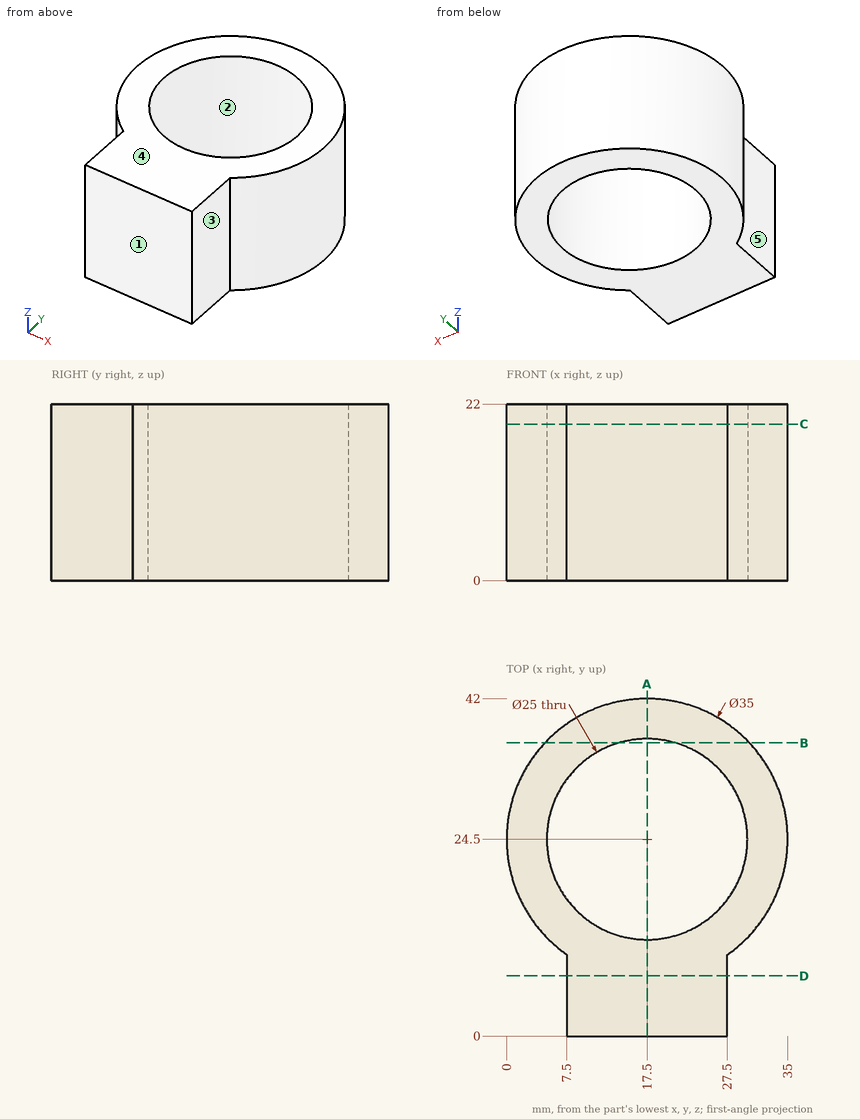
Verification items for this drawing (mm, ordinates from the low corner). A direction names the side the tool comes from. Coordinates: 2 decimals unless noted, no trailing zeros. Write each loop counter-clockwise with the first axis right and the second up, starting at its lowest first coordinate (ties: lowest second). Pieces come first, ordered by that corner, then holes. Notation, with made-up numbers: M 40.25,9 L 76.25,9 A14 ccw 76.25,17 Z; hole C 76,31 d10. An arc over 180 degrees is marked long. One line per item, written item: value. Start each with the question number.
(1) Sectioned sample at D-D, the plane y = 7.5. Enter the section's corners in (x, z).
(2) Sectioned sample at C-C, the plane z = 19.5. Enter the section's corners in (x, y).
(3) Tool access check on the marked faces 4 and 5. Record the directions out of +Z, -Z, +X, -X, +Y, -Y that give a thin tool (end or side, any length) a straight path to the whole face; none if there is none.
(4) Scan lines: line 1 along Y through (x, z) = (17.5, 17.5); line 2 along X through (y, z) = (2, 1.5); line 3 along Y through (x, z) = (21, 4.25). Record each from-to range of solid material in increasing order. Write a range as [from, to].
(5) Sectioned sample at A-A, the plane x = 17.5. Enter the section's corners in (y, z), and give its area (3 significant figures).
(6) Sectioned sample at B-B, the plane y = 36.5. Enter the section's corners in (x, z), and give its area (3 significant figures).
(7) Release check for a two-part mould opening along X. For the marked faces 1, 2 and 3 record: released by +X, released by -X, zero draft, split by the parting line, or undercut.
(8) Depth check by flat-ended pin: pin 1 (1 mm diameter, centred on y = 13, z = 7.5, fed in from -X); pin 2 (10 mm diameter, centred on x = 28, y = 18.5, fed in from +Z); pin 3 (5 mm diameter, centred on y = 6, z = 5.5, fed in from -X); pin 4 (11 mm diameter, centred on y = 3, z = 16, fed in from +X). Enter the tip coordinate at first touch or a pass-through.
Filled sheet:
1. outline: M 7.5,0 L 27.5,0 L 27.5,22 L 7.5,22 Z
2. outline: M 7.5,0 L 27.5,0 L 27.5,10.14 A17.5 ccw long 7.5,10.14 Z; hole C 17.5,24.5 d25
3. face 4: +Z, +X, -X, +Y, -Y
3. face 5: +Z, -Z, -X, -Y
4. line 1: [0, 12], [37, 42]
4. line 2: [7.5, 27.5]
4. line 3: [0, 12.5], [36.5, 41.65]
5. outline: M 0,0 L 12,0 L 12,22 L 0,22 Z; M 37,0 L 42,0 L 42,22 L 37,22 Z
5. area: 374 mm²
6. outline: M 4.76,0 L 14,0 L 14,22 L 4.76,22 Z; M 21,0 L 30.24,0 L 30.24,22 L 21,22 Z
6. area: 406 mm²
7. face 1: zero draft
7. face 2: undercut
7. face 3: released by +X
8. pin 1: x = 3.89
8. pin 2: z = 22
8. pin 3: x = 7.5
8. pin 4: x = 27.5
